```python
from build123d import *

# Parameters (mm, degrees)
ESQUISSE1_W                  = 30
ESQUISSE1_H                  = 35
BOSS_EXTRU_1_DEPTH           = 3
ESQUISSE2_R                  = 2
ENL_V_MAT_EXTRU_1_DEPTH      = 1
ENL_V_MAT_EXTRU_1_DEPTH_BACK = 4
ESQUISSE3_W                  = 30
ESQUISSE3_H                  = 6
BOSS_EXTRU_2_DEPTH           = 9.5
ESQUISSE4_R                  = 2.25
ENL_V_MAT_EXTRU_2_DEPTH      = 30
ENL_V_MAT_EXTRU_2_DEPTH_BACK = 7
BOSS_EXTRU_3_START           = -18
BOSS_EXTRU_3_DEPTH           = 6
CONG_1_R                     = 3
ESQUISSE6_R                  = 2.75
ENL_V_MAT_EXTRU_3_DEPTH      = 0.5


with BuildPart() as part:
    # Esquisse1 → Boss.-Extru.1 (new body)
    with BuildSketch(Plane.XY):
        with Locations((15, 17.5)):
            Rectangle(ESQUISSE1_W, ESQUISSE1_H)
    extrude(amount=BOSS_EXTRU_1_DEPTH)

    # Esquisse2 → Enlèv. mat.-Extru.1 (cut, two sides)
    with BuildSketch(Plane.XY.offset(3)) as enl_v_mat_extru_1_sk:
        with Locations((6, 25)):
            Circle(ESQUISSE2_R)
        with Locations((24, 25)):
            Circle(ESQUISSE2_R)
        with Locations((24, 13)):
            Circle(ESQUISSE2_R)
        with Locations((6, 13)):
            Circle(ESQUISSE2_R)
        with Locations((6, 19)):
            Circle(ESQUISSE2_R)
        with Locations((24, 19)):
            Circle(ESQUISSE2_R)
    extrude(amount=ENL_V_MAT_EXTRU_1_DEPTH, mode=Mode.SUBTRACT)
    extrude(enl_v_mat_extru_1_sk.sketch, amount=-ENL_V_MAT_EXTRU_1_DEPTH_BACK, mode=Mode.SUBTRACT)

    # Esquisse3 → Boss.-Extru.2 (add)
    with BuildSketch(Plane.XY.offset(3)):
        with Locations((15, 3)):
            Rectangle(ESQUISSE3_W, ESQUISSE3_H)
    extrude(amount=BOSS_EXTRU_2_DEPTH)

    # Esquisse4 → Enlèv. mat.-Extru.2 (cut, two sides)
    with BuildSketch(Plane(origin=(0, 6, 0), x_dir=(1, 0, 0), z_dir=(0, 1, 0))) as enl_v_mat_extru_2_sk:
        with Locations((25, -7.75)):
            Circle(ESQUISSE4_R)
        with Locations((5, -7.75)):
            Circle(ESQUISSE4_R)
    extrude(amount=ENL_V_MAT_EXTRU_2_DEPTH, mode=Mode.SUBTRACT)
    extrude(enl_v_mat_extru_2_sk.sketch, amount=-ENL_V_MAT_EXTRU_2_DEPTH_BACK, mode=Mode.SUBTRACT)

    # Esquisse5 → Boss.-Extru.3 (add)
    with BuildSketch(Plane(origin=(30, 0, 0), x_dir=(0, 0, -1), z_dir=(1, 0, 0)).offset(BOSS_EXTRU_3_START)):
        Polygon((-12.5, 6), (-3, 35), (-3, 6), align=None)
    extrude(amount=BOSS_EXTRU_3_DEPTH)

    # Congé1
    cong_1_edges = [part.edges().sort_by_distance(p)[0] for p in [
        (0, 3, 12.5),
        (30, 3, 12.5),
        (0, 35, 1.5),
        (30, 35, 1.5),
    ]]
    fillet(cong_1_edges, radius=CONG_1_R)

    # Esquisse6 → Enlèv. mat.-Extru.3 (cut)
    with BuildSketch(Plane.XY.offset(3)):
        with Locations((24, 25)):
            Circle(ESQUISSE6_R)
        with Locations((24, 19)):
            Circle(ESQUISSE6_R)
        with Locations((24, 13)):
            Circle(ESQUISSE6_R)
        with Locations((6, 13)):
            Circle(ESQUISSE6_R)
        with Locations((6, 19)):
            Circle(ESQUISSE6_R)
        with Locations((6, 25)):
            Circle(ESQUISSE6_R)
    extrude(amount=-ENL_V_MAT_EXTRU_3_DEPTH, mode=Mode.SUBTRACT)


solid = part.part
```
Model file for the job. Use its own axes, mm. A direction names the side the tool comes from. Coordinates: 2 decimals unless noted, no trailing zeros. Order: outer loops, then holes, each group sorted by start corner. A loop starts at its lowest first (then second) coordinate and runs counter-clockwise, first axis right, second up. Notation, with made-up numbers: (11.25, -37.75) - (27.25, -37.75) arc R31 ccw to (27.25, -13.75) - close; hole circle Ø6 at (-23, -16.75). An arc over 180 degrees is marked (long way). Return JSON: item names as keys, results as strings. Group by question number.
1) Flat gauge pins, fed straight in: P1, Ø6, axis at x = 5, z = 7.75, coming from the +Y side; P2, Ø7, axis at x = 24, y = 19, coming from the +Z side; P3, Ø4.5, axis at x = 6, y = 19, coming from the +Z side. Where does each tip first touch, or does it go through?
2) Tool access for faces 1 (the cylindrical face through (5.642, 27.727, 2.754)), 2 (the flat face through (15, 35, 1)): list every direction of +Z, -Z, +X, -X, +Y, -Y with a clear straight run to the whole face (end or side of a thin tool).
3) Saw through at A-A, the plane z = 7.75. Write the cut outline in (x, y), plus the area to 3 significant figures.
4) Saw through at B-B, the plane y = 3. Write the cut outline in (x, z).
5) Saw through at D-D, the plane x = 24. Count the separate pieces of the cut face and the enclosed holes in it, plus the area to 3 significant figures.
6) Probe line 1 (Y direction, x = 24, z = 0.6); line 2 (X direction, y = 2, z = 7.75); line 3 (Y direction, x = 6, z = 2.7). List the from-to ranges inside material, lowest first. Write a range as from..to.
7) Saw through at C-C, the plane y = 25. Write the cut outline in (x, z).
8) Mould opens along Y. For faces 3 (the flat face through (15, 0, 6)), 4 (the cylindrical face through (27.146, 3.042, 7.074)), 5 (the cylindrical face through (6, 21, 1)) say: released by +Y, released by -Y, zero draft, split by the parting line, or undercut.
Values found:
{
 "1": {"P1": "stops at y = 6", "P2": "stops at z = 3", "P3": "stops at z = 2.5"},
 "2": {"face 1": "+Z", "face 2": "+Z, -Z, +X, -X, +Y"},
 "3": {"outline": "(0, 0) - (2.75, 0) - (2.75, 6) - (0, 6) - close; (7.25, 0) - (22.75, 0) - (22.75, 6) - (18, 6) - (18, 20.5) - (12, 20.5) - (12, 6) - (7.25, 6) - close; (27.25, 0) - (30, 0) - (30, 6) - (27.25, 6) - close", "area": "213 mm²"},
 "4": {"outline": "(0, 0) - (30, 0) - (30, 9.5) arc R3 ccw to (27, 12.5) - (3, 12.5) arc R3 ccw to (0, 9.5) - close; hole circle Ø4.5 at (5, 7.75); hole circle Ø4.5 at (25, 7.75)"},
 "5": {"separate pieces": "5", "enclosed holes": "0", "area": "99.6 mm²"},
 "6": {"line 1": "y = 0..11, 15..17, 21..23, 27..35", "line 2": "x = 0..2.75, 7.25..22.75, 27.25..30", "line 3": "y = 0..10.25, 15.75..16.25, 21.75..22.25, 27.75..35"},
 "7": {"outline": "(0, 0) - (4, 0) - (4, 2.5) - (3.25, 2.5) - (3.25, 3) - (0, 3) - close; (8, 0) - (22, 0) - (22, 2.5) - (21.25, 2.5) - (21.25, 3) - (18, 3) - (18, 6.28) - (12, 6.28) - (12, 3) - (8.75, 3) - (8.75, 2.5) - (8, 2.5) - close; (26, 0) - (30, 0) - (30, 3) - (26.75, 3) - (26.75, 2.5) - (26, 2.5) - close"},
 "8": {"face 3": "released by -Y", "face 4": "zero draft", "face 5": "undercut"}
}
